Check sheet for the modelled part. Datum: model origin and axes. Units: mm. Face numbers are marked on the shaded views. A direction names the side the tool comes from. Coordinates: 2 decimals unless noted, no trailing zeros. Order: outer loops, then holes, each group sorted by start corner. A loop starts at its lowest first (then second) coordinate and runs counter-clockwise, first axis right, second up.
from build123d import *

# Parameters (mm, degrees)
SALIENTE_EXTRUIR2_DEPTH = 200
VACIADO2_T              = -3
CROQUIS6_R              = 8.2
CORTAR_EXTRUIR4_DEPTH   = 80
CROQUIS2_R              = 8.02
CORTAR_EXTRUIR5_DEPTH   = 3
CORTAR_EXTRUIR6_START   = -3
CROQUIS5_R              = 8.02
CORTAR_EXTRUIR6_DEPTH   = 3
CROQUIS7_W              = 7.4
CROQUIS7_H              = 7.4
CORTAR_EXTRUIR11_DEPTH  = 3
CROQUIS8_W              = 7.04
CROQUIS8_H              = 7.04
CORTAR_EXTRUIR12_DEPTH  = 3
CROQUIS9_W              = 35
CROQUIS9_H              = 35
CORTAR_EXTRUIR13_DEPTH  = 3
CROQUIS15_W             = 6
CROQUIS15_H             = 3
SALIENTE_EXTRUIR3_DEPTH = 75


with BuildPart() as part:
    # Croquis1 → Saliente-Extruir2 (new body)
    with BuildSketch(Plane(origin=(0, 0, 0), x_dir=(1, 0, 0), z_dir=(0, 1, 0))):
        Polygon((0, 0), (200, 0), (200, 80), (160, 80), align=None)
    extrude(amount=SALIENTE_EXTRUIR2_DEPTH)

    # Vaciado2
    vaciado2_openings = [part.faces().sort_by_distance(p)[0] for p in [
        (200, 100, -40),
    ]]
    offset(amount=VACIADO2_T, openings=vaciado2_openings, kind=Kind.INTERSECTION)

    # Croquis6 → Cortar-Extruir4 (cut)
    with BuildSketch(Plane(origin=(0, 0, 0), x_dir=(0, 0, -1), z_dir=(1, 0, 0))):
        with Locations(Location((30, 88.575, 0), (0, 0, 180))):
            Circle(CROQUIS6_R)
        with Locations(Location((30, 111.425, 0), (0, 0, 180))):
            Circle(CROQUIS6_R)
    extrude(amount=CORTAR_EXTRUIR4_DEPTH, mode=Mode.SUBTRACT)

    # Croquis2 → Cortar-Extruir5 (cut)
    with BuildSketch(Plane(origin=(0, 200, 0), x_dir=(1, 0, 0), z_dir=(0, 1, 0))):
        with Locations(Location((88.011571484, 15, 0), (0, 0, 270))):
            Circle(CROQUIS2_R)
        with Locations(Location((115.531571484, 15, 0), (0, 0, 270))):
            Circle(CROQUIS2_R)
    extrude(amount=-CORTAR_EXTRUIR5_DEPTH, mode=Mode.SUBTRACT)

    # Croquis5 → Cortar-Extruir6 (cut)
    with BuildSketch(Plane.XZ.offset(CORTAR_EXTRUIR6_START)):
        with Locations(Location((88.011571484, -15, 0), (0, 0, 90))):
            Circle(CROQUIS5_R)
        with Locations(Location((115.531571484, -15, 0), (0, 0, 90))):
            Circle(CROQUIS5_R)
    extrude(amount=CORTAR_EXTRUIR6_DEPTH, mode=Mode.SUBTRACT)

    # Croquis7 → Cortar-Extruir11 (cut)
    with BuildSketch(Plane.XY):
        with Locations((18.7, 13.7)):
            Rectangle(CROQUIS7_W, CROQUIS7_H)
    cortar_extruir11 = extrude(amount=-CORTAR_EXTRUIR11_DEPTH, mode=Mode.SUBTRACT)

    # Simetría5: Cortar-Extruir11 across plane
    add(cortar_extruir11.mirror(Plane.ZX.offset(100)), mode=Mode.SUBTRACT)

    # Croquis8 → Cortar-Extruir12 (cut)
    with BuildSketch(Plane.XY):
        with Locations((18.52, 100)):
            Rectangle(CROQUIS8_W, CROQUIS8_H)
    extrude(amount=-CORTAR_EXTRUIR12_DEPTH, mode=Mode.SUBTRACT)

    # Croquis9 → Cortar-Extruir13 (cut)
    with BuildSketch(Plane.XY):
        with Locations((174.5, 174.5)):
            Rectangle(CROQUIS9_W, CROQUIS9_H)
    cortar_extruir13 = extrude(amount=-CORTAR_EXTRUIR13_DEPTH, mode=Mode.SUBTRACT)

    # Simetría6: Cortar-Extruir13 across plane
    add(cortar_extruir13.mirror(Plane.ZX.offset(100)), mode=Mode.SUBTRACT)

    # Croquis15 → Saliente-Extruir3 (add)
    with BuildSketch(Plane(origin=(0, 0, -3), x_dir=(-1, 0, 0), z_dir=(0, 0, -1))):
        with Locations((-197, 4.5)):
            Rectangle(CROQUIS15_W, CROQUIS15_H)
    saliente_extruir3 = extrude(amount=SALIENTE_EXTRUIR3_DEPTH)

    # Simetría7: Saliente-Extruir3 across plane
    add(saliente_extruir3.mirror(Plane.ZX.offset(100)))

    # Croquis18 → Refrentado para tornillo tapón con cabeza plana de clavija de M33 (revolve, cut)
    with BuildSketch(Plane(origin=(196, 4, 0), x_dir=(0, -1, 0), z_dir=(1, 0, 0))):
        Polygon((0, 0), (0, 11.021463052), (1.7, 10), (1.7, 1.66), (3.36, 0), align=None)
    refrentado_para_tornillo_tap_n_con_cabez = revolve(axis=Axis((196, 4, 6.35), (0, 0, -1)), mode=Mode.SUBTRACT)

    # Simetría8: Refrentado para tornillo tapón con cabeza plana de clavija de M33 across plane
    add(refrentado_para_tornillo_tap_n_con_cabez.mirror(Plane.ZX.offset(100)), mode=Mode.SUBTRACT)

    # Simetría9: Refrentado para tornillo tapón con cabeza plana de clavija de M33 across plane
    add(refrentado_para_tornillo_tap_n_con_cabez.mirror(Plane(origin=(100, 0, 0), x_dir=(0, 0, 1), z_dir=(1, 0, 0))), mode=Mode.SUBTRACT)

    # Simetría9 copy 1 sketch → Simetría9 copy 1 (revolve, cut)
    with BuildSketch(Plane(origin=(4, 196, 0), x_dir=(0, 1, 0), z_dir=(-1, 0, 0))):
        Polygon((0, 0), (0, 11.021463052), (1.7, 10), (1.7, 1.66), (3.36, 0), align=None)
    revolve(axis=Axis((4, 196, 6.35), (0, 0, -1)), mode=Mode.SUBTRACT)

    # Partir1
    split(bisect_by=Plane.XY.offset(-3), keep=Keep.BOTTOM)


solid = part.part
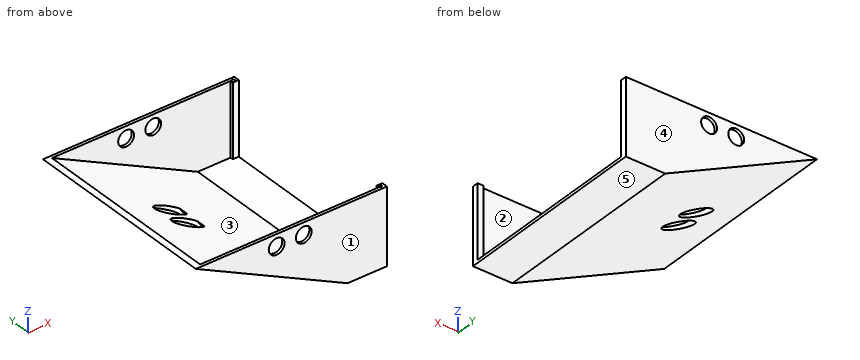
(1) Cross-section at B-B (x = 165.5). Enter the section's corners in (y, z), and give its area (3 significant figures).
Filled in:
outline: (0, -80) - (200, -80) - (200, -3) - (197, -3) - (197, -77) - (3, -77) - (3, -3) - (0, -3) - close
area: 1,040 mm2
(2) Go/stop test with flat-tipped pins: P1, Ø4, axis at x = 50.5, y = 62, coming from the -Z side; P2, Ø5, axis at x = 196, z = -37.5, coming from the -Y side; P3, Ø8, axis at x = 28, y = 117, coming from the -Z side; P4, Ø3.5, axis at y = 4.5, z = -26, coming from the -X side. Record where each tip stops, or that it passes through.
Filled in:
P1: stops at z = -26.25
P2: stops at y = 0
P3: stops at z = -16
P4: stops at x = 48.5
(3) Release check for a two-part mould opening along Y. For the marked faces 3, 4 and 5 record: +Y half, -Y half, draft (parallel to the pull), parting line (faces both ways), or undercut.
Filled in:
face 3: undercut
face 4: +Y half
face 5: draft
(4) Cross-section at D-D (y = 131.5). Enter the section's corners in (x, z).
Filled in:
outline: (6, -3) - (160, -80) - (200, -80) - (200, -77) - (160.71, -77) - (12.71, -3) - close
(5) Cross-section at A-A (z = -30). Enter the section's corners in (x, y) (3 decimals).
Filled in:
outline: (60, 0) - (200, 0) - (200, 6) - (194, 6) - (194, 3) - (66.708, 3) - (66.708, 80.375) - (60, 80.375) - close; (60, 96.775) - (66.708, 96.775) - (66.708, 103.225) - (60, 103.225) - close; (60, 119.625) - (66.708, 119.625) - (66.708, 197) - (194, 197) - (194, 194) - (200, 194) - (200, 200) - (60, 200) - close
(6) Thickness scan on probe 1 along Y at (x, z) = (152.5, -45.5); probe 2 along X at (y, z) = (0.75, -15); probe 3 along X at (y, z) = (4, -8). Record the ranges inside material, lowest first.
Filled in:
probe 1: y = 0 to 3, 197 to 200
probe 2: x = 30 to 79.99, 96.03 to 107.51, 123.55 to 200
probe 3: x = 16 to 22.71, 194 to 194.3, 197.7 to 200
(7) Tool access check on the marked faces 1 and 2. Record the directions out of +Z, -Z, +X, -X, +Y, -Y that give a thin tool (end or side, any length) a straight path to the whole face; none if there is none.
Filled in:
face 1: +Z, -Z, +X, -X, -Y
face 2: +Z
(8) Cross-section at C-C (z = -19). Enter the section's corners in (x, y).
Filled in:
outline: (38, 0) - (81.06, 0) - (81.06, 3) - (44.71, 3) - (44.71, 197) - (81.06, 197) - (81.06, 200) - (38, 200) - close; (94.96, 0) - (108.58, 0) - (108.58, 3) - (94.96, 3) - close; (94.96, 197) - (108.58, 197) - (108.58, 200) - (94.96, 200) - close; (122.48, 0) - (200, 0) - (200, 6) - (194, 6) - (194, 3) - (122.48, 3) - close; (122.48, 197) - (194, 197) - (194, 194) - (200, 194) - (200, 200) - (122.48, 200) - close
